from build123d import *

# Parameters (mm, degrees)
EXTRUDE_1_DEPTH     = 1.8
SKETCH_4_R          = 1.2835
CUT_EXTRUDE_1_DEPTH = 2.8


with BuildPart() as part:
    # 草图1 → 凸台-拉伸1 (new body)
    with BuildSketch(Plane(origin=(0, 0, 0), x_dir=(1, 0, 0), z_dir=(0, 1, 0))):
        Polygon((0, 3.175426481), (-2.75, 1.58771324), (-2.75, -1.58771324), (0, -3.175426481), (2.75, -1.58771324), (2.75, 1.58771324), align=None)
    extrude(amount=EXTRUDE_1_DEPTH)

    # 草图4 → 切除-拉伸1 (cut, through all)
    with BuildSketch(Plane(origin=(0, 1.8, 0), x_dir=(1, 0, 0), z_dir=(0, 1, 0))):
        Circle(SKETCH_4_R)
    extrude(amount=-CUT_EXTRUDE_1_DEPTH, mode=Mode.SUBTRACT)

    # 草图2 → 切除-旋转1 (revolve, cut)
    with BuildSketch(Plane(origin=(0, 0, 0), x_dir=(0, 0, -1), z_dir=(1, 0, 0))):
        Polygon((3.175426481, 1.8), (3.175426481, 1.554379907), (2.75, 1.8), align=None)
    revolve(axis=Axis((0, 0, 0), (0, 1, 0)), mode=Mode.SUBTRACT)

    # 草图3 → 切除-旋转2 (revolve, cut)
    with BuildSketch(Plane(origin=(0, 0, 0), x_dir=(0, 0, -1), z_dir=(1, 0, 0))):
        Polygon((3.175426481, 0), (3.175426481, 0.245620093), (2.75, 0), align=None)
    revolve(axis=Axis((0, 0, 0), (0, 1, 0)), mode=Mode.SUBTRACT)


solid = part.part
Verification items for the finished model (mm, model axes). Give positions to 0.01 mm unless a question says otherwise; leave off trailing zeros. Loops run counter-clockwise (first coordinate to the right, second up) from the corner with the lowest first, then second, coordinate; pieces in that order, holes last. Notation, with made-up numbers: (-18.5, 58) - (18.5, 58) arc R30 cw to (18.5, 90) - close; hole circle Ø11 at (68.25, 1.25). An arc over 180 degrees is marked (long way). Write each question's results on one line, items separated by ' | '.
1) Mould release check, pull along X, two halves, no side actions. Record for faces 1 (the conical face through (-2.51, 1.71, -1.46)), 2 (the flat face through (1.394, 0.887, -2.37)), 3 (the cylindrical face through (-0.278, 0.913, 1.253)): pulls with the +X half, pulls with the -X half, needs draft (parallel to the pull), parting line crosses it, or undercut.
Solution:
face 1: pulls with the -X half | face 2: pulls with the +X half | face 3: undercut
2) Material ranges on L1, parallel to X at y = 0.15, z = 0.25; L2, parallel to Z at x = 0.35, y = 1.35; L3, parallel to Z at x = 0.9, y = 1.5, recorded low to high. Write a range as from..to.
Solution:
L1: -2.75..-1.26, 1.26..2.75 | L2: -2.97..-1.23, 1.23..2.97 | L3: -2.66..-0.92, 0.92..2.66
3) Sectioned sample at A-A on y = 1.4. Record the boundary of the cut face in (x, z).
Solution:
outline: (-2.75, -1.59) - (0, -3.18) - (2.75, -1.59) - (2.75, 1.59) - (0, 3.18) - (-2.75, 1.59) - close; hole circle Ø2.57 at (0, 0)
